The model under review builds one solid part; all positions refer to its coordinate system, in mm. A direction names the side the tool comes from. Coordinates: 2 decimals unless noted, no trailing zeros. Write each loop counter-clockwise with the first axis right and the second up, starting at its lowest first coordinate (ties: lowest second). Pieces come first, ordered by that corner, then holes. Notation, with made-up numbers: (31, 18.25) - (88, 18.25) arc R21 cw to (88, 35.25) - close; hole circle Ø10 at (-36.5, 63). An arc over 180 degrees is marked (long way). Return JSON: item names as keys, results as strings. Group by question number.
(1) We need section A-A on x = -165. State the section outline as (y, z) points (3 decimals).
(2) We need section B-B on z = -21. State the section outline as (x, y) points (3 decimals).
(3) Tool access review of faces 1 (the face through (-576, 26, -47.625)), 2 (the face through (-1168.4, -0.5, -36.6)): name each direction out of +Z, -Z, +X, -X, +Y, -Y from which nothing blocks a thin tool from reaching the whole face with its end or side.
(4) For pin 1 Ø1 at (x, y) = (-842.5, 26) entering from +Z (3 decimals); pin 2 Ø4 at (x, y) = (-509.2, 37.57) entering from +Z; pin 3 Ø6 at (x, z) = (-520.7, -33.34) entering from +Y, all flat-tipped, find the tip position at first contact; note any pin that passes through.
(5) To check wall thickness, follow L1, parallel to Y at x = -1109, z = -48 (3 decimals); L2, parallel to Y at x = -123, z = -28 (3 decimals); L3, parallel to Z at x = -994, y = 44 (3 decimals). State the ranges of each line that lie inside material, in increasing order. Write a range as from..to.
```python
from build123d import *

# Parameters (mm, degrees)
F1_DEPTH = 1168.4
F2_R     = 2.6162
F3_DEPTH = 50.801
F4_R     = 2.6162
F5_DEPTH = 3.176
F6_R     = 2.6162
F7_DEPTH = 50.801


with BuildPart() as f1:
    # F0 (on Right) → F1 (new body)
    with BuildSketch(Plane.YZ):
        with BuildLine():
            Line((0, -44.45), (0, 0))
            Line((0, 0), (-3.175, 0))
            Line((-3.175, 0), (-3.175, -50.8))
            Line((-3.175, -50.8), (47.625, -50.8))
            Line((47.625, -50.8), (47.625, -47.625))
            Line((47.625, -47.625), (3.175, -47.625))
            ThreePointArc((3.175, -47.625), (0.929936, -46.695064), (0, -44.45))
        make_face()
    extrude(amount=-F1_DEPTH)

    # F2 (on face) → F3 (cut, through all)
    with BuildSketch(Plane(origin=(0, 0, -50.8), x_dir=(1, 0, 0), z_dir=(0, 0, -1))):
        with Locations((-1109.2, -6.8834)):
            Circle(F2_R)
        with Locations((-1109.2, -37.5666)):
            Circle(F2_R)
        with Locations((-959.2, -6.8834)):
            Circle(F2_R)
        with Locations((-959.2, -37.5666)):
            Circle(F2_R)
        with Locations((-809.2, -6.8834)):
            Circle(F2_R)
        with Locations((-809.2, -37.5666)):
            Circle(F2_R)
        with Locations((-659.2, -6.8834)):
            Circle(F2_R)
        with Locations((-659.2, -37.5666)):
            Circle(F2_R)
        with Locations((-509.2, -6.8834)):
            Circle(F2_R)
        with Locations((-509.2, -37.5666)):
            Circle(F2_R)
        with Locations((-359.2, -6.8834)):
            Circle(F2_R)
        with Locations((-359.2, -37.5666)):
            Circle(F2_R)
        with Locations((-209.2, -6.8834)):
            Circle(F2_R)
        with Locations((-209.2, -37.5666)):
            Circle(F2_R)
        with Locations((-59.2, -6.8834)):
            Circle(F2_R)
        with Locations((-59.2, -37.5666)):
            Circle(F2_R)
    extrude(amount=-F3_DEPTH, mode=Mode.SUBTRACT)

    # F4 (on face) → F5 (cut, through all)
    with BuildSketch(Plane.XY.offset(-47.625)):
        with Locations((-50.8, 22.225)):
            Circle(F4_R)
        with Locations((-1143, 22.225)):
            Circle(F4_R)
        with Locations((-1002.0681, 39.6875)):
            Circle(F4_R)
        with Locations((-191.7446, 39.6875)):
            Circle(F4_R)
    extrude(amount=-F5_DEPTH, mode=Mode.SUBTRACT)

    # F6 (on face) → F7 (cut, through all)
    with BuildSketch(Plane.XZ.offset(3.175)):
        with Locations((-368.3, -7.9375)):
            Circle(F6_R)
        with Locations((-215.9, -7.9375)):
            Circle(F6_R)
        with Locations((-520.7, -7.9375)):
            Circle(F6_R)
        with Locations((-520.7, -33.3375)):
            Circle(F6_R)
        with Locations((-368.3, -33.3375)):
            Circle(F6_R)
        with Locations((-215.9, -33.3375)):
            Circle(F6_R)
    extrude(amount=-F7_DEPTH, mode=Mode.SUBTRACT)


solid = f1.part
```
Ans:
{
 "1": {"outline": "(-3.175, -50.8) - (47.625, -50.8) - (47.625, -47.625) - (3.175, -47.625) arc R3.175 cw to (0, -44.45) - (0, 0) - (-3.175, 0) - close"},
 "2": {"outline": "(-1168.4, -3.175) - (0, -3.175) - (0, 0) - (-1168.4, 0) - close"},
 "3": {"face 1": "+Z, +X, -X, +Y", "face 2": "+Z, -Z, -X, +Y, -Y"},
 "4": {"pin 1": "z = -47.625", "pin 2": "through", "pin 3": "y = 0"},
 "5": {"L1": "-3.175..4.275, 9.492..34.958, 40.175..47.625", "L2": "-3.175..0", "L3": "-50.8..-47.625"}
}
